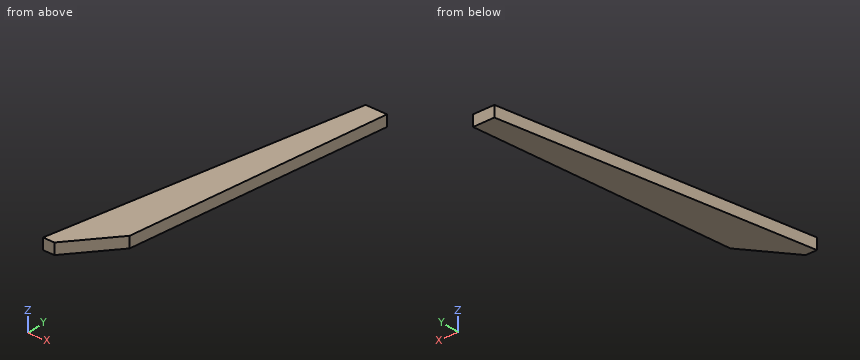
from build123d import *

# Parameters (mm, degrees)
BOSS_EXTRUDE1_DEPTH = 15
SCALE1_SCALE        = 0.6


with BuildPart() as part:
    # Sketch3 → Boss-Extrude1 (new body)
    with BuildSketch(Plane.XY):
        Polygon((400.577201165, 416), (361.233423479, 60.489600344), (311.944825715, 0), (296.597151769, 0), (371.734942748, 416), align=None)
    extrude(amount=BOSS_EXTRUDE1_DEPTH)


with BuildPart() as part_1:
    # Scale1: scaled about (353.237254905, 197.400686377, 7.5)
    add(part.part.scale(SCALE1_SCALE).moved(Location((141.294901962, 78.960274551, 3))))


solid = part_1.part
Check sheet for the modelled part. Datum: model origin and axes. Units: mm. Round coordinates to 2 decimals unless told otherwise and drop trailing zeros. Order: outer loops, then holes, each group sorted by start corner. A loop starts at its lowest first (then second) coordinate and runs counter-clockwise, first axis right, second up. Notation, with made-up numbers: M -6,63 L 24,63 A14 ccw 24,71 Z; hole C 9.25,14.25 d11. An arc over 180 degrees is marked long. One line per item, written item: value. Start each with the question number.
1. Section check B-B on y = 274.5. Enter the section's corners in (x, z).
2. Gauge pin test, flat end, axial feed: P1, Ø4, axis at y = 273, z = 7.5, coming from the +X side. Record the tip position at first contact, or that the pin passes through.
3. Scan lines: line 1 along X through (y, z) = (246, 11.25); line 2 along X through (y, z) = (196, 4.5). Record each from-to range of solid material in increasing order.
4. Section check A-A on z = 8.5. Enter the section's corners in (x, y), and give its area (3 significant figures).
5. Section check C-C on x = 348. Enter the section's corners in (y, z).
Results found:
1. outline: M 354.57,3 L 375.66,3 L 375.66,12 L 354.57,12 Z
2. P1: x = 375.71
3. line 1: 349.42 to 372.5
3. line 2: 340.39 to 366.97
4. outline: M 319.25,78.96 L 328.46,78.96 L 358.03,115.25 L 381.64,328.56 L 364.34,328.56 Z
4. area: 6,030 mm^2
5. outline: M 102.94,3 L 238.12,3 L 238.12,12 L 102.94,12 Z
